```python
from build123d import *

# Parameters (mm, degrees)
EXTRUDE_1_DEPTH     = 45
SKETCH_2_W          = 30
SKETCH_2_H          = 35
CUT_EXTRUDE_1_DEPTH = 40.5
SKETCH_4_R          = 2.65
CUT_EXTRUDE_2_DEPTH = 40
SKETCH_5_W          = 35
SKETCH_5_H          = 29
CUT_EXTRUDE_3_DEPTH = 25
SKETCH_6_R          = 2.65
CUT_EXTRUDE_4_DEPTH = 97.566039579
SKETCH_7_W          = 55
SKETCH_7_H          = 3
CUT_EXTRUDE_5_DEPTH = 97.566039579
FILLET_1_R          = 3


with BuildPart() as part:
    # 草图1 → 凸台-拉伸1 (new body)
    with BuildSketch(Plane.XY):
        Polygon((25, 0), (-25, 0), (-25, -10), (-80, -10), (-80, -20), (-60, -20), (-60, -40), (60, -40), (60, -20), (80, -20), (80, -10), (25, -10), align=None)
    extrude(amount=EXTRUDE_1_DEPTH)

    # 草图2 → 切除-拉伸1 (cut)
    with BuildSketch(Plane(origin=(0, 0, 0), x_dir=(-1, 0, 0), z_dir=(0, 0, -1))):
        with Locations((0, -22.5)):
            Rectangle(SKETCH_2_W, SKETCH_2_H)
    extrude(amount=-CUT_EXTRUDE_1_DEPTH, mode=Mode.SUBTRACT)

    # 草图4 → 切除-拉伸2 (cut)
    with BuildSketch(Plane.XZ.offset(5)):
        with Locations((0, 18.8)):
            Circle(SKETCH_4_R)
    extrude(amount=-CUT_EXTRUDE_2_DEPTH, mode=Mode.SUBTRACT)

    # 草图5 → 切除-拉伸3 (cut)
    with BuildSketch(Plane.XZ.offset(40)):
        with Locations((-37.5, 22.5)):
            Rectangle(SKETCH_5_W, SKETCH_5_H)
        with Locations((37.5, 22.5)):
            Rectangle(SKETCH_5_W, SKETCH_5_H)
    extrude(amount=-CUT_EXTRUDE_3_DEPTH, mode=Mode.SUBTRACT)

    # 草图6 → 切除-拉伸4 (cut, through all)
    with BuildSketch(Plane(origin=(0, -10, 0), x_dir=(1, 0, 0), z_dir=(0, 1, 0))):
        with Locations(Location((70, -10, 0), (0, 0, 180))):
            Circle(SKETCH_6_R)
        with Locations(Location((70, -35, 0), (0, 0, 180))):
            Circle(SKETCH_6_R)
        with Locations(Location((-70, -35, 0), (0, 0, 180))):
            Circle(SKETCH_6_R)
        with Locations(Location((-70, -10, 0), (0, 0, 270))):
            Circle(SKETCH_6_R)
    extrude(amount=-CUT_EXTRUDE_4_DEPTH, mode=Mode.SUBTRACT)

    # 草图7 → 切除-拉伸5 (cut, through all)
    with BuildSketch(Plane(origin=(0, -10, 0), x_dir=(1, 0, 0), z_dir=(0, 1, 0))):
        with Locations((-52.5, -1.5)):
            Rectangle(SKETCH_7_W, SKETCH_7_H)
        with Locations((-52.5, -43.5)):
            Rectangle(SKETCH_7_W, SKETCH_7_H)
        with Locations((52.5, -43.5)):
            Rectangle(SKETCH_7_W, SKETCH_7_H)
        with Locations((52.5, -1.5)):
            Rectangle(SKETCH_7_W, SKETCH_7_H)
    extrude(amount=-CUT_EXTRUDE_5_DEPTH, mode=Mode.SUBTRACT)

    # 圆角1
    fillet_1_edges = [part.edges().sort_by_distance(p)[0] for p in [
        (80, -10, 22.5),
        (-80, -10, 22.5),
        (0, 0, 0),
        (-25, 0, 22.5),
        (0, 0, 45),
        (25, 0, 22.5),
        (25, -25, 42),
        (-25, -25, 42),
        (-25, -10, 22.5),
        (-25, -25, 3),
        (25, -25, 3),
        (25, -10, 22.5),
        (-37.5, -15, 37),
        (-20, -15, 22.5),
        (-37.5, -15, 8),
        (-55, -15, 22.5),
        (-55, -27.5, 37),
        (-20, -27.5, 37),
        (-20, -27.5, 8),
        (-55, -27.5, 8),
        (20, -27.5, 37),
        (37.5, -15, 37),
        (55, -27.5, 37),
        (55, -15, 22.5),
        (20, -15, 22.5),
        (20, -27.5, 8),
        (55, -27.5, 8),
        (37.5, -15, 8),
    ]]
    fillet(fillet_1_edges, radius=FILLET_1_R - 0.0001)  # a hair under: the kernel refuses the full size


solid = part.part
```
CAD build for the part. Positions are in the model's coordinates, mm. A direction names the side the tool comes from. Round coordinates to 2 decimals unless told otherwise and drop trailing zeros. Loops run counter-clockwise (first coordinate to the right, second up) from the corner with the lowest first, then second, coordinate; pieces in that order, holes last. Notation, with made-up numbers: M 67.25,-30 L 104.25,-30 A35 cw 104.25,4 Z; hole C 19.5,-24 d5. An arc over 180 degrees is marked long. Return JSON: item names as keys, results as strings. Group by question number.
(1) Saw through at B-B, the plane x = -70. List the corners of the cut face in (y, z), and give its area (3 significant figures).
(2) Saw through at D-D, the plane x = 35.5. List the corners of the cut face in (y, z).
(3) Wall check: probe 1 along Z at (x, y) = (70, -17); probe 2 along X at (y, z) = (-18.5, 28.5); probe 3 along X at (y, z) = (-36.5, 16). Give the ranges that are in metal, low to high. Write a range as [from, to].
(4) Tool access for faces 4 (the flat face through (-60, -30, 22)), 5 (the cylindrical face through (-37.3, -15.86, 36.1)), 6 (the flat face through (48, -25, 3)), 7 (the flat face through (15, -23, 20)): list every direction of +Z, -Z, +X, -X, +Y, -Y with a clear straight run to the whole face (end or side of a thin tool).
(5) Saw through at A-A, the plane x = 0. List the corners of the cut face in (y, z), and give its area (3 significant figures).
(6) Drop flat-ended pins along their axis: P1, Ø5, axis at x = 47, z = 19.5, coming from the -Y side; P2, Ø5, axis at x = -41.5, y = -7, coming from the -Z side; P3, Ø10, axis at y = -33.5, z = 26.5, coming from the -X side; P4, Ø9, axis at x = 60, y = -18, coming from the -Z side. Give the stop position or say it passes through.
(7) Mould opens along Z. For faces 1 (the flat face through (-49, -21, 42)), 2 (the cylindrical face through (67.472, -14.93, 10.796)), 3 (the flat face through (-80, -16, 22)) say: +Z half, -Z half, draft (parallel to the pull), parting line (faces both ways), or undercut.
Answer list:
{
 "1": {"outline": "M -20,3 L -10,3 L -10,7.35 L -20,7.35 Z; M -20,12.65 L -10,12.65 L -10,32.35 L -20,32.35 Z; M -20,37.65 L -10,37.65 L -10,42 L -20,42 Z", "area": "284 mm2"},
 "2": {"outline": "M -40,3 L -10,3 L -10,42 L -40,42 L -40,37 L -18,37 A3 cw -15,34 L -15,11 A3 cw -18,8 L -40,8 Z"},
 "3": {"probe 1": "[3, 7.35], [12.65, 32.35], [37.65, 42]", "probe 2": "[-80, -55], [-20, -15], [15, 20], [55, 80]", "probe 3": "[-60, -55], [-20, -15], [15, 20], [55, 60]"},
 "4": {"face 4": "+Z, -Z, -X, -Y", "face 5": "-Y", "face 6": "-Z, +X, +Y, -Y", "face 7": "-Z, -Y"},
 "5": {"outline": "M -40,40.5 L -5,40.5 L -5,21.45 L 0,21.45 L 0,42 A3 ccw -3,45 L -40,45 Z; M -5,0 L -3,0 A3 ccw 0,3 L 0,16.15 L -5,16.15 Z", "area": "352 mm2"},
 "6": {"P1": "y = -15", "P2": "through", "P3": "x = -60", "P4": "z = 3"},
 "7": {"face 1": "+Z half", "face 2": "undercut", "face 3": "draft"}
}
